Geometry: final body of the model. Coordinates: model frame, mm. A direction names the side the tool comes from. Give positions to 0.01 mm unless a question says otherwise; leave off trailing zeros. Loops run counter-clockwise (first coordinate to the right, second up) from the corner with the lowest first, then second, coordinate; pieces in that order, holes last.
```python
from build123d import *

# Parameters (mm, degrees)
F0_R     = 11.3
F1_DEPTH = 7.9
F3_DEPTH = 3.55
F4_R     = 2.75
F5_DEPTH = 5.35


with BuildPart() as f1:
    # F0 (on Front) → F1 (new body)
    with BuildSketch(Plane.XZ):
        Circle(F0_R)
    extrude(amount=F1_DEPTH)

    # F2 (on Front) → F3 (join)
    with BuildSketch(Plane.XZ):
        Polygon((-3.75, 6.495191), (-7.5, 0), (-3.75, -6.495191), (3.75, -6.495191), (7.5, 0), (3.75, 6.495191), align=None)
    extrude(amount=-F3_DEPTH)

    # F4 (on face) → F5 (join)
    with BuildSketch(Plane(origin=(0, 3.55, 0), x_dir=(-1, 0, 0), z_dir=(0, 1, 0))):
        Circle(F4_R)
    extrude(amount=F5_DEPTH)


solid = f1.part
```
Q1. Section query A-A, the plane x = 0. Return loops of the section in (y, z).
Q2. Reachability of faces 1 (the face through (0, 2, 6.495)), 2 (the face through (0.596, 6.188, -2.685)), 3 (the face through (-5.651, 1.75, -3.202)) from +Z, -Z, +X, -X, +Y, -Y: full face, straight path, thin tool, end or side. Return the list, or none.
Q3. Section query C-C, the plane y = 7.5. Return loops of the section in (x, z), and give its area (3 significant figures).
Q4. Section query B-B, the plane z = 1.5. Return loops of the section in (x, y), and give its area (3 significant figures).
Q5. Material intervals for probe 1 along Y at (x, z) = (5, -6.5); probe 2 along Y at (x, z) = (5.5, -2.5); probe 3 along X at (y, z) = (-3.25, -0.5), sorted ascending.
Q6. Pin query (flat end, axial travel): pin 1 Ø10 at (y, z) = (1.5, -6.5) entering from +X; pin 2 Ø3 at (x, y) = (2, 0) entering from +Z; pin 3 Ø1.5 at (x, y) = (-3.5, -1) entering from +Z. Return the tip coordinate at first contact, or that it passes through.
Q7. Section query D-D, the plane x = 5.5. Return loops of the section in (y, z).
Resolved:
1. outline: (-7.9, -11.3) - (0, -11.3) - (0, -6.5) - (3.55, -6.5) - (3.55, -2.75) - (8.9, -2.75) - (8.9, 2.75) - (3.55, 2.75) - (3.55, 6.5) - (0, 6.5) - (0, 11.3) - (-7.9, 11.3) - close
2. face 1: +Z, +X, -X, +Y
2. face 2: +Y
2. face 3: -Z, -X, +Y
3. outline: circle Ø5.5 at (0, 0)
3. area: 23.8 mm2
4. outline: (-11.2, -7.9) - (11.2, -7.9) - (11.2, 0) - (6.63, 0) - (6.63, 3.55) - (2.3, 3.55) - (2.3, 8.9) - (-2.3, 8.9) - (-2.3, 3.55) - (-6.63, 3.55) - (-6.63, 0) - (-11.2, 0) - close
4. area: 249 mm2
5. probe 1: y = -7.9 to 0
5. probe 2: y = -7.9 to 3.55
5. probe 3: x = -11.29 to 11.29
6. pin 1: stops at x = 11.17
6. pin 2: stops at z = 11.29
6. pin 3: stops at z = 10.96
7. outline: (-7.9, -9.87) - (0, -9.87) - (0, -3.46) - (3.55, -3.46) - (3.55, 3.46) - (0, 3.46) - (0, 9.87) - (-7.9, 9.87) - close
